For this review, take the finished solid that the model builds, in its own axes (mm). A direction names the side the tool comes from. Round coordinates to 2 decimals unless told otherwise and drop trailing zeros. Order: outer loops, then holes, each group sorted by start corner. A loop starts at its lowest first (then second) coordinate and runs counter-clockwise, first axis right, second up. Notation, with made-up numbers: (8.5, -16.5) - (55.5, -16.5) arc R18 cw to (55.5, -5.5) - close; hole circle Ø7 at (-14.5, -15.75). An arc over 180 degrees is marked (long way). Write each question's results on one line, items separated by ' | '. Start each with the question number.
(1) Take a section at B-B, the plane y = 3. Give the boundary of the cut face in (x, z), plus the area to 3 significant figures.
(2) For L1, parallel to X at y = 0.8, z = 14; L2, parallel to X at y = 25, z = -12; L3, parallel to Z at x = 10.9, y = 18, list the stretches that pass through material, from the lowest coordinate up. Write a range as from..to.
(3) Take a section at A-A, the plane z = 0. Give the boundary of the cut face in (x, y), plus the area to 3 significant figures.
(4) Insertion check: pin 1 Ø10 at (y, z) = (24.5, -9) entering from +X; pin 2 Ø4 at (x, z) = (16.5, -14) entering from -Y; pin 3 Ø10 at (y, z) = (17, -9) entering from -X; pin 4 Ø4.5 at (x, z) = (0, 0) entering from -Y. Each pin has a flat end and moves straight along its axis. Give the tip position at first contact, or say it passes through.
(5) For faces 5 (the flat face through (10, 13, 4)), 6 (the flat face through (-11.5, 26, 0)), 7 (the cylindrical face through (-19.68, 0.74, -16.02)), 8 (the flat face through (11.5, 10, 0)), list the 3-axis set-ups (+Z, -Z, +X, -X, +Y, -Y) from which the entire face can be reached by the end or side of a thin tool; tool diameter is ignored.
(6) Draft analysis for pull direction X (two halves, no side actions). For faces 1 (the flat face through (-10.3, 20.2, -19)), 2 (the flat face through (14.453, 0.74, -18.245)), 3 (the cylindrical face through (17.51, 0.74, -15.11)), 4 (the flat face through (-10, 13, 4)), state which applies: pulls with the +X half, pulls with the -X half, needs draft (parallel to the pull), parting line crosses it, or undercut.
(7) Take a section at C-C, the plane z = 4. Give the boundary of the cut face in (x, y), plus the area to 3 significant figures.
(8) Take a section at D-D, the plane y = 21. Give the boundary of the cut face in (x, z), plus the area to 3 significant figures.
```python
from build123d import *

# Parameters (mm, degrees)
BOSS_EXTRUDE1_DEPTH = 19
SKETCH4_R           = 2
CUT_EXTRUDE1_DEPTH  = 1.5
FILLET1_R           = 0.3
FILLET2_R           = 0.3
FILLET3_R           = 0.3
SKETCH3_R           = 1.5
BOSS_EXTRUDE2_DEPTH = 1.5
SKETCH7_R           = 6
CUT_EXTRUDE2_DEPTH  = 52.088159098


with BuildPart() as part:
    # Sketch1 → Boss-Extrude1 (new, symmetric)
    with BuildSketch(Plane.XY):
        Polygon((-10, 0), (-10, 33.5), (10, 33.5), (10, 0), (11.5, 0), (11.5, 35), (-11.5, 35), (-11.5, 0), align=None)
    extrude(amount=BOSS_EXTRUDE1_DEPTH, both=True)

    # Sketch4 → Cut-Extrude1 (cut)
    with BuildSketch(Plane(origin=(0, 35, 0), x_dir=(1, 0, 0), z_dir=(0, 1, 0))):
        with Locations(Location((0, 0, 0), (0, 0, 270))):
            Circle(SKETCH4_R)
    extrude(amount=-CUT_EXTRUDE1_DEPTH, mode=Mode.SUBTRACT)

    # Fillet1
    fillet1_edges = [part.edges().sort_by_distance(p)[0] for p in [
        (-10, 0, 0),
    ]]
    fillet(fillet1_edges, radius=FILLET1_R)

    # Fillet2
    fillet2_edges = [part.edges().sort_by_distance(p)[0] for p in [
        (10, 0, 0),
    ]]
    fillet(fillet2_edges, radius=FILLET2_R)

    # Fillet3
    fillet3_edges = [part.edges().sort_by_distance(p)[0] for p in [
        (-11.5, 35, 0),
        (11.5, 35, 0),
    ]]
    fillet(fillet3_edges, radius=FILLET3_R)

    # Sketch3 → Boss-Extrude2 (add)
    # profile 1 of 2: a face of its own
    with BuildSketch(Plane(origin=(0, 0, 0), x_dir=(1, 0, 0), z_dir=(0, 1, 0))):
        with BuildLine():
            ThreePointArc((-17.49039307, -17.469121771), (-19.659238221, -16.047079248), (-20.5, -13.593670627))
            Line((-20.5, -13.593670627), (-20.5, 13.593670627))
            ThreePointArc((-20.5, 13.593670627), (-19.659238221, 16.047079248), (-17.49039307, 17.469121771))
            Line((-17.49039307, 17.469121771), (-11.5, 19))
            Line((-11.5, 19), (-11.5, -19))
            Line((-11.5, -19), (-17.49039307, -17.469121771))
        make_face()
        with Locations(Location((-16.5, -14, 0), (0, 0, 270))):
            Circle(SKETCH3_R, mode=Mode.SUBTRACT)
        with Locations(Location((-16.5, 14, 0), (0, 0, 270))):
            Circle(SKETCH3_R, mode=Mode.SUBTRACT)
    # profile 2 of 2: a face of its own
    with BuildSketch(Plane(origin=(0, 0, 0), x_dir=(1, 0, 0), z_dir=(0, 1, 0))):
        with BuildLine():
            Line((17.49039307, -17.469121771), (11.5, -19))
            Line((11.5, -19), (11.5, 19))
            Line((11.5, 19), (17.49039307, 17.469121771))
            ThreePointArc((17.49039307, 17.469121771), (19.659238221, 16.047079248), (20.5, 13.593670627))
            Line((20.5, 13.593670627), (20.5, -13.593670627))
            ThreePointArc((20.5, -13.593670627), (19.659238221, -16.047079248), (17.49039307, -17.469121771))
        make_face()
        with Locations(Location((16.5, -14, 0), (0, 0, 270))):
            Circle(SKETCH3_R, mode=Mode.SUBTRACT)
        with Locations(Location((16.5, 14, 0), (0, 0, 270))):
            Circle(SKETCH3_R, mode=Mode.SUBTRACT)
    extrude(amount=BOSS_EXTRUDE2_DEPTH)

    # Sketch7 → Cut-Extrude2 (cut, through all)
    with BuildSketch(Plane.ZY.offset(11.5)):
        with Locations(Location((0, 18, 0), (0, 0, 270))):
            Circle(SKETCH7_R)
    extrude(amount=-CUT_EXTRUDE2_DEPTH, mode=Mode.SUBTRACT)


solid = part.part
```
Results below:
1) outline: (-11.5, -19) - (-10, -19) - (-10, 19) - (-11.5, 19) - close; (10, -19) - (11.5, -19) - (11.5, 19) - (10, 19) - close | area: 114 mm^2
2) L1: x = -20.48..-18, -15..-10, 10..15, 18..20.48 | L2: x = -11.5..-10, 10..11.5 | L3: z = -19..-6, 6..19
3) outline: (-20.5, 0) - (-10.3, 0) arc R0.3 ccw to (-10, 0.3) - (-10, 12) - (-11.5, 12) - (-11.5, 1.5) - (-20.5, 1.5) - close; (-11.5, 24) - (-10, 24) - (-10, 33.5) - (-2, 33.5) - (-2, 35) - (-11.2, 35) arc R0.3 ccw to (-11.5, 34.7) - close; (2, 33.5) - (10, 33.5) - (10, 24) - (11.5, 24) - (11.5, 34.7) arc R0.3 ccw to (11.2, 35) - (2, 35) - close; (10, 0.3) arc R0.3 ccw to (10.3, 0) - (20.5, 0) - (20.5, 1.5) - (11.5, 1.5) - (11.5, 12) - (10, 12) - close | area: 120 mm^2
4) pin 1: stops at x = 11.5 | pin 2: stops at y = 0 | pin 3: stops at x = -11.5 | pin 4: stops at y = 33.5
5) face 5: +Z, -Z, -Y | face 6: +Z, -Z, -X, +Y | face 7: -Z, -X, +Y, -Y | face 8: +Z, -Z, +X, +Y
6) face 1: needs draft | face 2: pulls with the +X half | face 3: undercut | face 4: undercut
7) outline: (-20.5, 0) - (-10.3, 0) arc R0.3 ccw to (-10, 0.3) - (-10, 13.53) - (-11.5, 13.53) - (-11.5, 1.5) - (-20.5, 1.5) - close; (-11.5, 22.47) - (-10, 22.47) - (-10, 33.5) - (10, 33.5) - (10, 22.47) - (11.5, 22.47) - (11.5, 34.7) arc R0.3 ccw to (11.2, 35) - (-11.2, 35) arc R0.3 ccw to (-11.5, 34.7) - close; (10, 0.3) arc R0.3 ccw to (10.3, 0) - (20.5, 0) - (20.5, 1.5) - (11.5, 1.5) - (11.5, 13.53) - (10, 13.53) - close | area: 135 mm^2
8) outline: (-11.5, -19) - (-10, -19) - (-10, -5.2) - (-11.5, -5.2) - close; (-11.5, 5.2) - (-10, 5.2) - (-10, 19) - (-11.5, 19) - close; (10, -19) - (11.5, -19) - (11.5, -5.2) - (10, -5.2) - close; (10, 5.2) - (11.5, 5.2) - (11.5, 19) - (10, 19) - close | area: 82.8 mm^2
